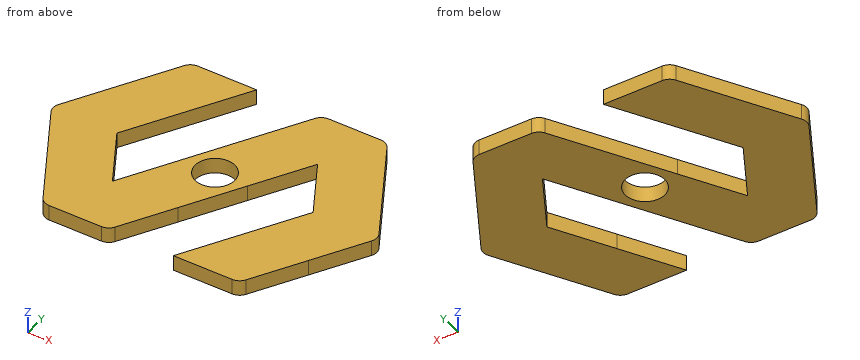
from build123d import *

# Parameters (mm, degrees)
F2_DEPTH = 4
F3_D     = 10.2
F4_R     = 3


with BuildPart() as f2:
    # F0 (on Top) → F2 (new body)
    with BuildSketch(Plane.XY):
        Polygon((8.5, 14.7224318643), (0, 0), (17, 0), (25.5, 14.7224318643), (34, 29.4448637287), (25.5, 44.167295593), (17, 58.8897274573), (0, 58.8897274573), (-8.5, 44.167295593), (-17, 29.4448637287), (-25.5, 14.7224318643), (-34, 29.4448637287), (-25.5, 44.167295593), (-17, 58.8897274573), (-34, 58.8897274573), (-42.5, 44.167295593), (-51, 29.4448637287), (-42.5, 14.7224318643), (-34, 0), (-17, 0), (-8.5, 14.7224318643), (0, 29.4448637287), (8.5, 44.167295593), (17, 29.4448637287), align=None)
    extrude(amount=F2_DEPTH)

    # F3 (through all)
    with Locations(Plane(origin=(0, 0, 0), x_dir=(1, 0, 0), z_dir=(0, 0, -1))):
        with Locations((-8.5, -29.4448637287)):
            Hole(F3_D / 2)

    # F4
    f4_edges = [f2.edges().sort_by_distance(p)[0] for p in [
        (-51, 29.444864, 2),
        (-34, 58.889727, 2),
        (0, 58.889727, 2),
        (17, 58.889727, 2),
        (34, 29.444864, 2),
        (17, 0, 2),
        (-17, 0, 2),
        (-34, 0, 2),
    ]]
    fillet(f4_edges, radius=F4_R)


solid = f2.part
Build history of the part. All positions in model axes, mm. Round coordinates to 2 decimals unless told otherwise and drop trailing zeros. Write each loop counter-clockwise with the first axis right and the second up, starting at its lowest first coordinate (ties: lowest second). Pieces come first, ordered by that corner, then holes. Notation, with made-up numbers: (26, 62.25) -> (47, 62.25) arc R21 ccw to (47, 80.25) -> close; hole circle Ø11 at (-10.5, 7.5). An arc over 180 degrees is marked (long way). Write item = value, one per line.
(1) Band-saw the part on A-A (y = 42). Give the cut face in (x, z), then the cut area to 3 significant figures.
Answer:
outline = (-43.75, 0) -> (-26.75, 0) -> (-26.75, 4) -> (-43.75, 4) -> close; (-9.75, 0) -> (7.25, 0) -> (7.25, 4) -> (-9.75, 4) -> close; (9.75, 0) -> (26.75, 0) -> (26.75, 4) -> (9.75, 4) -> close
area = 204 mm2
(2) Probe L1, parallel to Y at x = -8.5, z = 3.1; L2, parallel to X at y = 25, z = 2.7; L3, parallel to X at y = 41, z = 1.15. List the from-to ranges inside material, lowest first.
Answer:
L1 = 14.72 to 24.34, 34.54 to 44.17
L2 = -48.43 to -31.43, -19.57 to -11, -6 to -2.57, 14.43 to 31.43
L3 = -44.33 to -27.33, -10.33 to 6.67, 10.33 to 27.33
(3) Band-saw the part on D-D (x = -39). Give the cut face in (y, z), then the cut area to 3 significant figures.
Answer:
outline = (8.66, 0) -> (50.23, 0) -> (50.23, 4) -> (8.66, 4) -> close
area = 166 mm2
(4) Band-saw the part on B-B (z = 1.4). Give the cut face in (x, y).
Answer:
outline = (-50.13, 27.94) -> (-34.87, 1.5) arc R3 ccw to (-32.27, 0) -> (-18.73, 0) arc R3 ccw to (-16.13, 1.5) -> (8.5, 44.17) -> (17, 29.44) -> (0, 0) -> (15.27, 0) arc R3 ccw to (17.87, 1.5) -> (33.13, 27.94) arc R3 ccw to (33.13, 30.94) -> (17.87, 57.39) arc R3 ccw to (15.27, 58.89) -> (1.73, 58.89) arc R3 ccw to (-0.87, 57.39) -> (-25.5, 14.72) -> (-34, 29.44) -> (-17, 58.89) -> (-32.27, 58.89) arc R3 ccw to (-34.87, 57.39) -> (-50.13, 30.94) arc R3 ccw to start; hole circle Ø10.2 at (-8.5, 29.44)
(5) Band-saw the part on C-C (y = 54). Give the cut face in (x, z), then the cut area to 3 significant figures.
Answer:
outline = (-36.82, 0) -> (-19.82, 0) -> (-19.82, 4) -> (-36.82, 4) -> close; (-2.82, 0) -> (19.82, 0) -> (19.82, 4) -> (-2.82, 4) -> close
area = 159 mm2
(6) Flat gauge pin, fed straight in: pin 1 (2 mm diameter, centred on y = 39, z = 2, fed in from +X). Where does the tip first touch, or does it go through?
Answer:
pin_1 = 29.06
